Geometry: final body of the model. Coordinates: model frame, mm. A direction names the side the tool comes from. Coordinates: 2 decimals unless noted, no trailing zeros. Write each loop counter-clockwise with the first axis right and the second up, starting at its lowest first coordinate (ties: lowest second). Pieces come first, ordered by that corner, then holes. Notation, with made-up numbers: (21, 54) -> (76, 54) arc R13 cw to (76, 76) -> close; hole circle Ø1 at (45.25, -23). An arc over 180 degrees is marked (long way). One line per item, written item: value. Start each with the question number.
from build123d import *

# Parameters (mm, degrees)
SKICA1_R                      = 2.25
SKICA1_R_2                    = 1.75
SKICA1_W                      = 20.4
SKICA1_H                      = 5.2
SKICA1_H_2                    = 5.3
P_IDAT_VYSUNUT_M1_DEPTH       = 10
SKICA2_W                      = 20.6
SKICA2_H                      = 10.95
ODEBRAT_VYSUNUT_M1_DEPTH      = 1.2
SKICA4_R                      = 1.85
ODEBRAT_VYSUNUT_M2_DEPTH      = 69.460937767
ODEBRAT_VYSUNUT_M3_DEPTH      = 69.625505463
ODEBRAT_VYSUNUT_M3_DEPTH_BACK = 69.625505463
SKICA5_W                      = 18.35
SKICA5_H                      = 23.35
SKICA5_3_W                    = 20.95
SKICA5_3_H                    = 25.95
ODEBRAT_VYSUNUT_M4_DEPTH      = 1.2
SKICA6_R                      = 1
ODEBRAT_VYSUNUT_M5_DEPTH      = 1.2
SKICA7_R                      = 1
ODEBRAT_VYSUNUT_M6_DEPTH      = 69.625505463
ZAOBLIT3_R                    = 2
ZAOBLIT4_R                    = 1
ZAOBLIT5_R                    = 1
ZAOBLIT6_R                    = 1


with BuildPart() as part:
    # Skica1 → Přidat vysunutím1 (new body)
    with BuildSketch(Plane.XY):
        Polygon((-57.5, 36.1), (57.5, 36.1), (57.5, 17.95), (17.5, 17.95), (17.5, 0), (-17.5, 0), (-17.5, 6.1), (-57.5, 6.1), align=None)
        with Locations((-52.5, 31.1)):
            Circle(SKICA1_R, mode=Mode.SUBTRACT)
        with Locations((-22.5, 31.1)):
            Circle(SKICA1_R, mode=Mode.SUBTRACT)
        with Locations((-52.5, 11.1)):
            Circle(SKICA1_R, mode=Mode.SUBTRACT)
        with Locations((-22.5, 11.1)):
            Circle(SKICA1_R, mode=Mode.SUBTRACT)
        with Locations((-52.5, 21.1)):
            Circle(SKICA1_R_2, mode=Mode.SUBTRACT)
        with Locations((-22.5, 21.1)):
            Circle(SKICA1_R_2, mode=Mode.SUBTRACT)
        with Locations((0, 8.6)):
            Rectangle(SKICA1_W, SKICA1_H, mode=Mode.SUBTRACT)
        with Locations((0, 24.75)):
            Rectangle(SKICA1_W, SKICA1_H_2, mode=Mode.SUBTRACT)
    extrude(amount=-P_IDAT_VYSUNUT_M1_DEPTH)

    # Skica2 → Odebrat vysunutím1 (cut)
    with BuildSketch(Plane.XY):
        with Locations((37.5, 23.425)):
            Rectangle(SKICA2_W, SKICA2_H)
    extrude(amount=-ODEBRAT_VYSUNUT_M1_DEPTH, mode=Mode.SUBTRACT)

    # Skica4 → Odebrat vysunutím2 (cut, through all)
    with BuildSketch(Plane.XY.offset(-1.2)):
        with Locations((45.5, 26.35)):
            Circle(SKICA4_R)
        with Locations((29.5, 26.35)):
            Circle(SKICA4_R)
    extrude(amount=-ODEBRAT_VYSUNUT_M2_DEPTH, mode=Mode.SUBTRACT)

    # Skica5 → Odebrat vysunutím3 (cut, two sides: drawn at the far end of the back side and taken through both)
    with BuildSketch(Plane.XY.offset(-ODEBRAT_VYSUNUT_M3_DEPTH_BACK)):
        with Locations((-37.5, 21.1)):
            Rectangle(SKICA5_W, SKICA5_H)
    extrude(amount=ODEBRAT_VYSUNUT_M3_DEPTH + ODEBRAT_VYSUNUT_M3_DEPTH_BACK, mode=Mode.SUBTRACT)

    # Skica5<3> → Odebrat vysunutím4 (cut)
    with BuildSketch(Plane.XY):
        with Locations((-37.5, 21.1)):
            Rectangle(SKICA5_3_W, SKICA5_3_H)
    extrude(amount=-ODEBRAT_VYSUNUT_M4_DEPTH, mode=Mode.SUBTRACT)

    # Skica6 → Odebrat vysunutím5 (cut)
    with BuildSketch(Plane.XY):
        with Locations((-47.975, 34.075)):
            Circle(SKICA6_R)
        with Locations((-27.025, 34.075)):
            Circle(SKICA6_R)
        with Locations((-47.975, 8.125)):
            Circle(SKICA6_R)
        with Locations((-27.025, 8.125)):
            Circle(SKICA6_R)
        with Locations((27.2, 28.9)):
            Circle(SKICA6_R)
        with Locations((47.8, 28.9)):
            Circle(SKICA6_R)
    extrude(amount=-ODEBRAT_VYSUNUT_M5_DEPTH, mode=Mode.SUBTRACT)

    # Skica7 → Odebrat vysunutím6 (cut, through all)
    with BuildSketch(Plane.XY):
        with Locations((-10.2, 27.4)):
            Circle(SKICA7_R)
        with Locations((-10.2, 22.1)):
            Circle(SKICA7_R)
        with Locations((10.2, 22.1)):
            Circle(SKICA7_R)
        with Locations((10.2, 27.4)):
            Circle(SKICA7_R)
        with Locations((-10.2, 11.2)):
            Circle(SKICA7_R)
        with Locations((-10.2, 6)):
            Circle(SKICA7_R)
        with Locations((10.2, 6)):
            Circle(SKICA7_R)
        with Locations((10.2, 11.2)):
            Circle(SKICA7_R)
    extrude(amount=-ODEBRAT_VYSUNUT_M6_DEPTH, mode=Mode.SUBTRACT)

    # Zaoblit3
    zaoblit3_edges = [part.edges().sort_by_distance(p)[0] for p in [
        (17.5, 0, -5),
        (-17.5, 0, -5),
        (-57.5, 6.1, -5),
        (-57.5, 36.1, -5),
        (57.5, 36.1, -5),
        (57.5, 17.95, -5),
    ]]
    fillet(zaoblit3_edges, radius=ZAOBLIT3_R)

    # Zaoblit4
    zaoblit4_edges = [part.edges().sort_by_distance(p)[0] for p in [
        (-17.5, 6.1, -5),
        (17.5, 17.95, -5),
    ]]
    fillet(zaoblit4_edges, radius=ZAOBLIT4_R)

    # Zaoblit5
    zaoblit5_edges = [part.edges().sort_by_distance(p)[0] for p in [
        (-46.675, 32.775, -5.6),
        (-28.325, 32.775, -5.6),
        (-28.325, 9.425, -5.6),
        (-46.675, 9.425, -5.6),
        (46.8, 28.9, -0.6),
        (47.8, 27.9, -0.6),
        (-28.025, 34.075, -0.6),
        (-27.025, 33.075, -0.6),
        (-47.975, 9.125, -0.6),
        (-46.975, 8.125, -0.6),
        (-27.025, 9.125, -0.6),
        (-28.025, 8.125, -0.6),
        (27.2, 27.9, -0.6),
        (28.2, 28.9, -0.6),
        (-47.975, 33.075, -0.6),
        (-46.975, 34.075, -0.6),
        (27.2, 17.95, -0.6),
        (47.8, 17.95, -0.6),
    ]]
    fillet(zaoblit5_edges, radius=ZAOBLIT5_R)

    # Zaoblit6
    zaoblit6_edges = [part.edges().sort_by_distance(p)[0] for p in [
        (10.2, 23.1, -5),
        (10.2, 26.4, -5),
        (10.2, 10.2, -5),
        (10.2, 7, -5),
        (-9.2, 6, -5),
        (-10.2, 10.2, -5),
        (-9.2, 22.1, -5),
        (-10.2, 26.4, -5),
        (-9.2, 11.2, -5),
        (9.2, 27.4, -5),
        (9.2, 22.1, -5),
        (-10.2, 23.1, -5),
        (-10.2, 7, -5),
        (9.2, 6, -5),
        (9.2, 11.2, -5),
        (-9.2, 27.4, -5),
    ]]
    fillet(zaoblit6_edges, radius=ZAOBLIT6_R)


solid = part.part
Q1. Access query for faces 1 (the flat face through (0, 0, -5)), 2 (the flat face through (-38, 32.775, -6)), 3 (the flat face through (-37, 6.1, -5)). Directions: +Z, -Z, +X, -X, +Y, -Y. A direction counts if a zero-diameter tool reaches every point of the face in a straight line with its end or side. Return the directions, or none.
Q2. Line query: L1, parallel to X at y = 24, z = -8.5 (3 decimals); L2, parallel to Y at x = -22.5, z = -4.5; L3, parallel to Y at x = -10, z = -3. Output: solid intervals per line, ascending. Write a range as from..to.
Q3. Cut plane B-B on z = -4. Count the separate pieces of the cut face and the enclosed holes in it, and give its area (3 significant figures).
Q4. Cut plane A-A on x = -40.5. Output: boundary loops of the cut face in (y, z) (3 decimals).
Q5. First-contact query: P1, Ø5, axis at x = -34, z = -6, coming from the -Y side; P2, Ø2.5, axis at x = 10.2, y = 22.1, coming from the +Z side; P3, Ø0.6, axis at y = 15.5, z = -0.5, coming from the +X side; P4, Ø1.6, axis at x = -47.975, y = 34.075, coming from the +Z side. Flat tips, straight axial feed; report the tip coordinate or a pass-through.
Q6. Draft query along Y for faces 4 (the cylindrical face through (-54.16, 32.62, -4.93)), 5 (the flat face through (1, 18, -10)), 6 (the cylindrical face through (-16.93, 0.6, -5.07)). Return one class per face: pulls with the +Y half, pulls with the -Y half, needs draft (parallel to the pull), parting line crosses it, or undercut.
Solution:
1. face 1: +Z, -Z, +X, -X, -Y
1. face 2: +Z, -Z
1. face 3: +Z, -Z, -X, -Y
2. L1: -57.5..-46.675, -28.325..-10.2, 10.2..57.5
2. L2: 6.1..8.85, 13.35..19.35, 22.85..28.85, 33.35..36.1
2. L3: 0..5.02, 12.18..21.12, 28.38..36.1
3. separate pieces: 1
3. enclosed holes: 11
3. area: 2,420 mm²
4. outline: (6.1, -10) -> (9.425, -10) -> (9.425, -1.2) -> (8.125, -1.2) -> (8.125, 0) -> (6.1, 0) -> close; (32.775, -10) -> (36.1, -10) -> (36.1, 0) -> (34.075, 0) -> (34.075, -1.2) -> (32.775, -1.2) -> close
5. P1: y = 6.1
5. P2: z = 0
5. P3: x = 17.5
5. P4: z = -1.2
6. face 4: undercut
6. face 5: needs draft
6. face 6: pulls with the -Y half
